Could you check a few things on this drawing? It's one solid part, dimensions in mm from its lowest x, y, z. Give positions to 0.01 mm unless a question says otherwise; leave off trailing zeros. Order: outer loops, then holes, each group sorted by start corner. A loop starts at its lowest first (then second) coordinate and runs counter-clockwise, first axis right, second up.
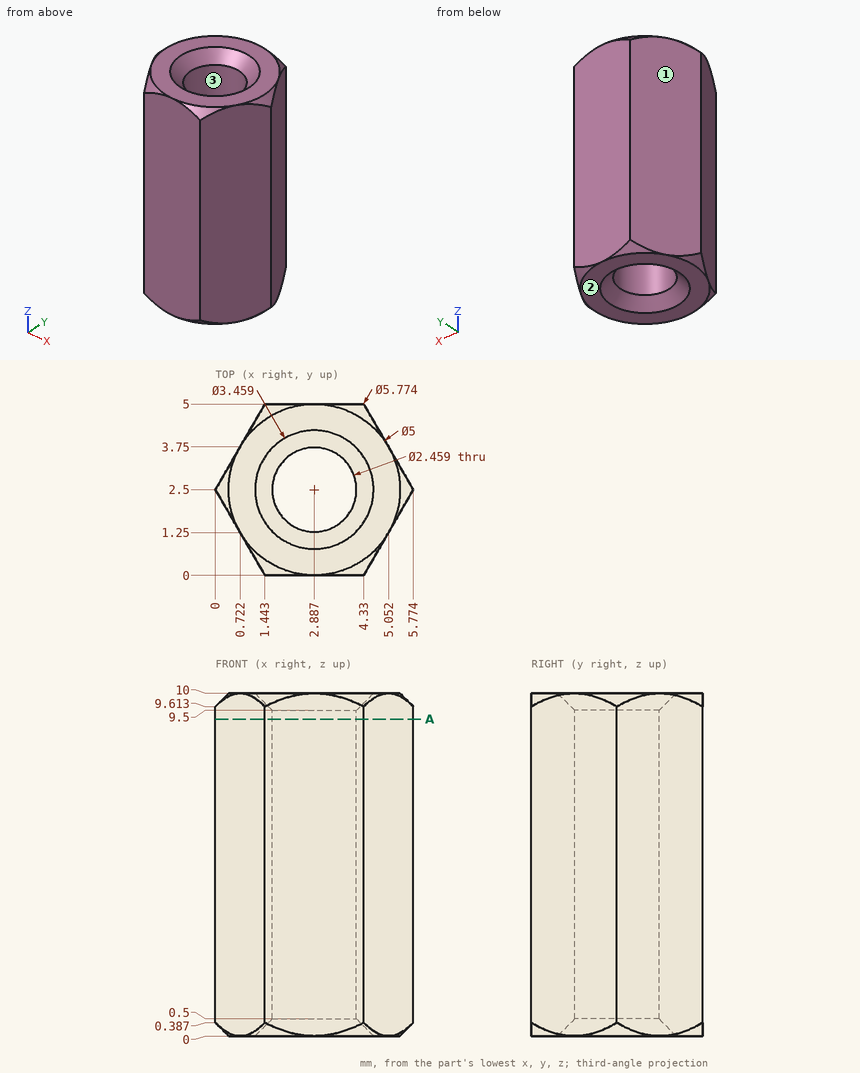
Q1. If we section it at A-A on z = 9.25: List the corners of the cut face in (x, y) for me.
Filled sheet:
outline: (0, 2.5) - (1.44, 0) - (4.33, 0) - (5.77, 2.5) - (4.33, 5) - (1.44, 5) - close; hole circle Ø2.46 at (2.89, 2.5)
Q2. Thinking about a two-plate mould opening in X: for the marked faces 1, 2 and 3, which applies, released by +X, released by -X, zero draft, split by the parting line, or undercut?
Filled sheet:
face 1: released by -X
face 2: zero draft
face 3: undercut
Q3. I'm going to push flat-ended pins straight in: P1, Ø1.5, axis at y = 3, z = 2.5, coming from the -X side; P2, Ø1.5, axis at y = 4, z = 3.5, coming from the +X side; P3, Ø1.5, axis at y = 4, z = 3.5, coming from the -X side. Where does each tip first touch, or does it pass through?
Filled sheet:
P1: stops at x = 0
P2: stops at x = 5.34
P3: stops at x = 0.43
Q4. I need wall thicknesses on L1, parallel to Y at x = 2.45, z = 6; L2, parallel to X at y = 3.3, z = 3.5 (1 decimal); L3, parallel to X at y = 1.95, z = 8 (1 decimal). Which ranges of each line are inside material? Lowest first, please.
Filled sheet:
L1: y = 0 to 1.35, 3.65 to 5
L2: x = 0.5 to 2, 3.8 to 5.3
L3: x = 0.3 to 1.8, 4 to 5.5
